Here's how the part is built. I have some questions about the finished solid (model axes, mm). Face numbers are marked on the shaded views. A direction names the side the tool comes from. Give positions to 0.01 mm unless a question says otherwise; leave off trailing zeros. Loops run counter-clockwise (first coordinate to the right, second up) from the corner with the lowest first, then second, coordinate; pieces in that order, holes last. Notation, with made-up numbers: (57.5, -19.5) - (79.5, -19.5) arc R22 ccw to (79.5, -6.5) - close; hole circle Ø7 at (85, 83.5). An arc over 180 degrees is marked (long way). Use a Markdown table: item, result.
from build123d import *

# Parameters (mm, degrees)
F0_W      = 279.4
F0_H      = 76.2
F0_W_2    = 266.7
F0_H_2    = 63.5
F1_DEPTH  = 38.1
F2_W      = 279.4
F2_H      = 76.2
F3_DEPTH  = 6.35
F4_W      = 63.5
F4_H      = 38.1
F5_DEPTH  = 25
F6_W      = 279.4
F6_H      = 76.2
F7_DEPTH  = 127
F8_W      = 279.4
F8_H      = 76.2
F8_W_2    = 266.7
F8_H_2    = 63.5
F9_DEPTH  = 38.1
F10_W     = 63.5
F10_H     = 38.1
F11_DEPTH = 25
F12_W     = 279.4
F12_H     = 76.2
F13_DEPTH = 6.35
F14_R     = 2.5
F15_DEPTH = 6.35
F16_R     = 2.5
F17_DEPTH = 6.35


with BuildPart() as f1:
    # F0 (on Top) → F1 (new body)
    with BuildSketch(Plane.XY):
        Rectangle(F0_W, F0_H)
        Rectangle(F0_W_2, F0_H_2, mode=Mode.SUBTRACT)
    extrude(amount=F1_DEPTH)

    # F2 (on face) → F3 (join)
    with BuildSketch(Plane(origin=(0, 0, 0), x_dir=(1, 0, 0), z_dir=(0, 0, -1))):
        Rectangle(F2_W, F2_H)
    extrude(amount=F3_DEPTH)

    # F4 (on face) → F5 (cut)
    with BuildSketch(Plane(origin=(133.35, 0, 0), x_dir=(0, -1, 0), z_dir=(-1, 0, 0))):
        with Locations((0, 19.05)):
            Rectangle(F4_W, F4_H)
    extrude(amount=-F5_DEPTH, mode=Mode.SUBTRACT)

    # F6 (on face) → F7 (join)
    with BuildSketch(Plane.XY.offset(38.1)):
        Rectangle(F6_W, F6_H)
    extrude(amount=F7_DEPTH)

    # F8 (on face) → F9 (join)
    with BuildSketch(Plane.XY.offset(165.1)):
        Rectangle(F8_W, F8_H)
        Rectangle(F8_W_2, F8_H_2, mode=Mode.SUBTRACT)
    extrude(amount=F9_DEPTH)

    # F10 (on face) → F11 (cut)
    with BuildSketch(Plane(origin=(133.35, 0, 0), x_dir=(0, -1, 0), z_dir=(-1, 0, 0))):
        with Locations((0, 184.15)):
            Rectangle(F10_W, F10_H)
    extrude(amount=-F11_DEPTH, mode=Mode.SUBTRACT)

    # F12 (on face) → F13 (join)
    with BuildSketch(Plane.XY.offset(203.2)):
        Rectangle(F12_W, F12_H)
    extrude(amount=F13_DEPTH)

    # F14 (on face) → F15 (cut, through all)
    with BuildSketch(Plane.XY.offset(209.55)):
        with Locations((101.6, 25.4)):
            Circle(F14_R)
        with Locations((101.6, -25.4)):
            Circle(F14_R)
        with Locations((-101.6, 25.4)):
            Circle(F14_R)
        with Locations((-101.6, -25.4)):
            Circle(F14_R)
    extrude(amount=-F15_DEPTH, mode=Mode.SUBTRACT)

    # F16 (on face) → F17 (cut, through all)
    with BuildSketch(Plane(origin=(0, 0, -6.35), x_dir=(1, 0, 0), z_dir=(0, 0, -1))):
        with Locations((-101.6, -25.4)):
            Circle(F16_R)
        with Locations((-101.6, 25.4)):
            Circle(F16_R)
        with Locations((101.6, -25.4)):
            Circle(F16_R)
        with Locations((101.6, 25.4)):
            Circle(F16_R)
    extrude(amount=-F17_DEPTH, mode=Mode.SUBTRACT)


solid = f1.part
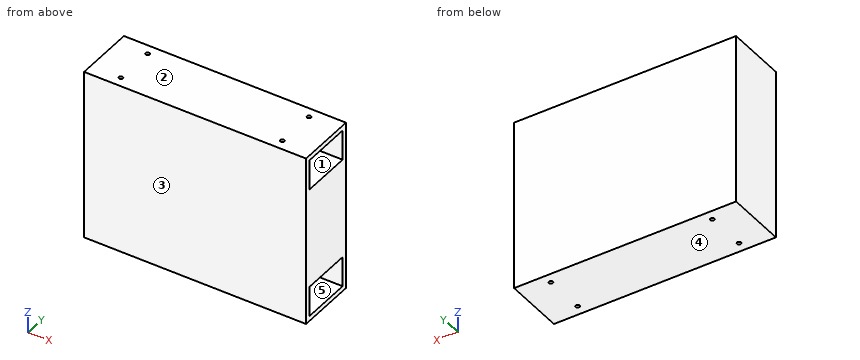
(1) Suppose I cut it at A-A on y = -6. Write out the boundary of the cut face in (x, z).
A:
| item | result |
|---|---|
| outline | (-139.7, -6.35) - (139.7, -6.35) - (139.7, 0) - (-133.35, 0) - (-133.35, 38.1) - (139.7, 38.1) - (139.7, 165.1) - (-133.35, 165.1) - (-133.35, 203.2) - (139.7, 203.2) - (139.7, 209.55) - (-139.7, 209.55) - close |
(2) Suppose I cut it at C-C on x = 49.5. Write out the boundary of the cut face in (y, z).
A:
| item | result |
|---|---|
| outline | (-38.1, -6.35) - (38.1, -6.35) - (38.1, 209.55) - (-38.1, 209.55) - close; hole (-31.75, 0) - (31.75, 0) - (31.75, 38.1) - (-31.75, 38.1) - close; hole (-31.75, 165.1) - (31.75, 165.1) - (31.75, 203.2) - (-31.75, 203.2) - close |
(3) Will these pins go through, and if not, where does the flat tip stop? pin 1 (3 mm diameter, centred on y = 22, z = 176, fed in from +X); pin 2 (4 mm diameter, centred on x = 101.6, y = 25.4, fed in from -Z); pin 3 (3 mm diameter, centred on x = -101.6, y = 25.4, fed in from +Z).
A:
| item | result |
|---|---|
| pin 1 | x = -133.35 |
| pin 2 | z = 38.1 |
| pin 3 | z = 165.1 |
(4) On a 3-axis mill with a long thin cutter (end or side, diameter ignored), from which of +Z, -Z, +X, -X, +Y, -Y can I reach the whole of each face in a straight line? I mean the marked faces 1 and 2. Say none if no direction works.
A:
| item | result |
|---|---|
| face 1 | +X |
| face 2 | +Z, +X, -X, +Y, -Y |
(5) If I drill on line 1 (Z direction, x = -108.5, y = 23); line 2 (X direction, y = 25.4, z = -4); line 3 (Y direction, x = 101.6, z = 206.25), over which ranges is the centre line in solid material (lowest first)?
A:
| item | result |
|---|---|
| line 1 | -6.35 to 0, 38.1 to 165.1, 203.2 to 209.55 |
| line 2 | -139.7 to -104.1, -99.1 to 99.1, 104.1 to 139.7 |
| line 3 | -38.1 to -27.9, -22.9 to 22.9, 27.9 to 38.1 |
(6) We'd pull the mould along Y, two halves only. Please class the marked faces 3, 4 and 5: pulls with the +Y half, pulls with the -Y half, needs draft (parallel to the pull), parting line crosses it, or undercut.
A:
| item | result |
|---|---|
| face 3 | pulls with the -Y half |
| face 4 | needs draft |
| face 5 | undercut |
(7) Suppose I cut it at B-B on z = 31. Write out the boundary of the cut face in (x, y).
A:
| item | result |
|---|---|
| outline | (-139.7, -38.1) - (139.7, -38.1) - (139.7, -31.75) - (-133.35, -31.75) - (-133.35, 31.75) - (139.7, 31.75) - (139.7, 38.1) - (-139.7, 38.1) - close |
